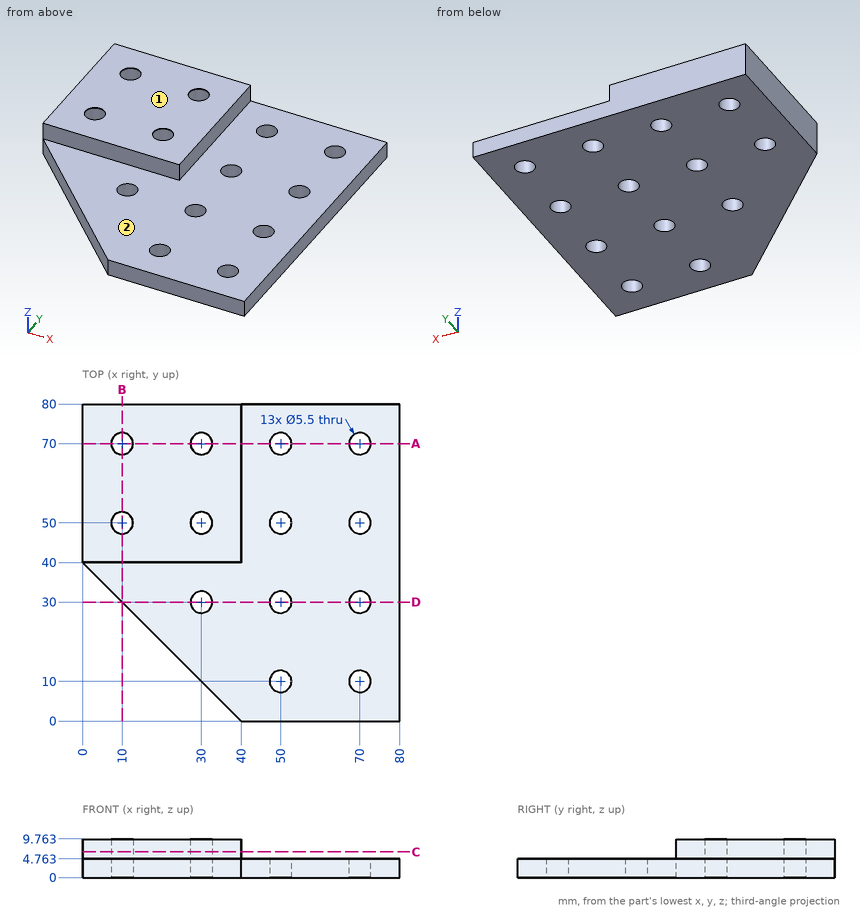
Design review of the part shown in the three views and the two pictorial views. Dimensions are in mm from the part's minimum x, y and z. A direction names the side the tool comes from. Give positions to 0.01 mm unless a question says otherwise; leave off trailing zeros. Order: outer loops, then holes, each group sorted by start corner. A loop starts at its lowest first (then second) coordinate and runs counter-clockwise, first axis right, second up. Notation, with made-up numbers: M 61,59 L 103,59 A28 ccw 103,95 Z; hole C -32,88 d4. An arc over 180 degrees is marked long. Answer in a Markdown table with one row per item. Add a question column.
(1) For the marked faces 1 and 2, list the 3-axis set-ups (+Z, -Z, +X, -X, +Y, -Y) from which the entire face can be reached by the end or side of a thin tool; tool diameter is ignored.
(2) Consider section A-A on y = 70. State the section outline as (x, z) points, and give its area (3 significant figures).
(3) Consider section B-B on x = 10. State the section outline as (y, z) points, and give its area (3 significant figures).
(4) Wall thickness on probe 1 along Y at (x, z) = (70, 1.75); probe 2 along X at (y, z) = (70, 6.75); probe 3 along X at (y, z) = (48.5, 4.25) (1 decimal): over which ranges is each line inside the solid? List them lowest first. Write a range as [from, to].
(5) For pin 1 (7 mm diameter, centred on x = 10, y = 70, fed in from +Z); pin 2 (7 mm diameter, centred on x = 50, y = 10, fed in from +Z); pin 3 (2.5 mm diameter, centred on y = 69, z = 7.5, fed in from +X), all flat-tipped, find the tip position at first contact; note any pin that passes through.
(6) Consider section C-C on z = 6.5. State the section outline as (x, y) points.
(7) Consider section D-D on y = 30. State the section outline as (x, z) points.
Evaluation:
| question | item | result |
|---|---|---|
| 1 | face 1 | +Z, +X, -X, +Y, -Y |
| 1 | face 2 | +Z, +X, -Y |
| 2 | outline | M 0,0 L 7.25,0 L 7.25,9.76 L 0,9.76 Z; M 12.75,0 L 27.25,0 L 27.25,9.76 L 12.75,9.76 Z; M 32.75,0 L 47.25,0 L 47.25,4.76 L 40,4.76 L 40,9.76 L 32.75,9.76 Z; M 52.75,0 L 67.25,0 L 67.25,4.76 L 52.75,4.76 Z; M 72.75,0 L 80,0 L 80,4.76 L 72.75,4.76 Z |
| 2 | area | 421 mm^2 |
| 3 | outline | M 30,0 L 47.25,0 L 47.25,9.76 L 40,9.76 L 40,4.76 L 30,4.76 Z; M 52.75,0 L 67.25,0 L 67.25,9.76 L 52.75,9.76 Z; M 72.75,0 L 80,0 L 80,9.76 L 72.75,9.76 Z |
| 3 | area | 331 mm^2 |
| 4 | probe 1 | y = [0, 7.25], [12.75, 27.25], [32.75, 47.25], [52.75, 67.25], [72.75, 80] |
| 4 | probe 2 | x = [0, 7.25], [12.75, 27.25], [32.75, 40] |
| 4 | probe 3 | x = [0, 7.7], [12.3, 27.7], [32.3, 47.7], [52.3, 67.7], [72.3, 80] |
| 5 | pin 1 | stops at z = 9.76 |
| 5 | pin 2 | stops at z = 4.76 |
| 5 | pin 3 | stops at x = 40 |
| 6 | outline | M 0,40 L 40,40 L 40,80 L 0,80 Z; hole C 10,50 d5.5; hole C 10,70 d5.5; hole C 30,50 d5.5; hole C 30,70 d5.5 |
| 7 | outline | M 10,0 L 27.25,0 L 27.25,4.76 L 10,4.76 Z; M 32.75,0 L 47.25,0 L 47.25,4.76 L 32.75,4.76 Z; M 52.75,0 L 67.25,0 L 67.25,4.76 L 52.75,4.76 Z; M 72.75,0 L 80,0 L 80,4.76 L 72.75,4.76 Z |
